Could you check a few things on this model? Use its own coordinates, in mm. Face numbers are marked on the shaded views. A direction names the side the tool comes from. Give positions to 0.01 mm unless a question says otherwise; leave off trailing zeros. Write each loop counter-clockwise with the first axis right and the second up, starting at its lowest first coordinate (ties: lowest second). Pieces come first, ordered by that corner, then holes. Notation, with made-up numbers: (47.25, 56) -> (94.25, 56) arc R17 ccw to (94.25, 69) -> close; hole circle Ø6 at (86.25, 69). An arc over 180 degrees is marked (long way). One line per question, with ' | ' between items.
from build123d import *

# Parameters (mm, degrees)
SKETCH1_W           = 70
SKETCH1_H           = 70
BOSS_EXTRUDE1_DEPTH = 10
CUT_EXTRUDE1_DEPTH  = 51.497524692


with BuildPart() as part:
    # Sketch1 → Boss-Extrude1 (new body)
    with BuildSketch(Plane(origin=(0, 0, 0), x_dir=(1, 0, 0), z_dir=(0, 1, 0))):
        Rectangle(SKETCH1_W, SKETCH1_H)
    extrude(amount=BOSS_EXTRUDE1_DEPTH)

    # Sketch4 → Cut-Extrude1 (cut, through all)
    with BuildSketch(Plane(origin=(0, 10, 0), x_dir=(1, 0, 0), z_dir=(0, 1, 0))):
        with BuildLine():
            Line((-26.870057685, 3.25), (-18.384776311, 3.25))
            ThreePointArc((-18.384776311, 3.25), (-15.134776311, 0), (-18.384776311, -3.25))
            Line((-18.384776311, -3.25), (-26.870057685, -3.25))
            ThreePointArc((-26.870057685, -3.25), (-30.120057685, 0), (-26.870057685, 3.25))
        make_face()
        with BuildLine():
            Line((3.25, 26.870057685), (3.25, 18.384776311))
            ThreePointArc((3.25, 18.384776311), (0, 15.134776311), (-3.25, 18.384776311))
            Line((-3.25, 18.384776311), (-3.25, 26.870057685))
            ThreePointArc((-3.25, 26.870057685), (0, 30.120057685), (3.25, 26.870057685))
        make_face()
        with BuildLine():
            Line((26.870057685, -3.25), (18.384776311, -3.25))
            ThreePointArc((18.384776311, -3.25), (15.134776311, 0), (18.384776311, 3.25))
            Line((18.384776311, 3.25), (26.870057685, 3.25))
            ThreePointArc((26.870057685, 3.25), (30.120057685, 0), (26.870057685, -3.25))
        make_face()
        with BuildLine():
            Line((-3.25, -26.870057685), (-3.25, -18.384776311))
            ThreePointArc((-3.25, -18.384776311), (0, -15.134776311), (3.25, -18.384776311))
            Line((3.25, -18.384776311), (3.25, -26.870057685))
            ThreePointArc((3.25, -26.870057685), (0, -30.120057685), (-3.25, -26.870057685))
        make_face()
    extrude(amount=-CUT_EXTRUDE1_DEPTH, mode=Mode.SUBTRACT)


solid = part.part
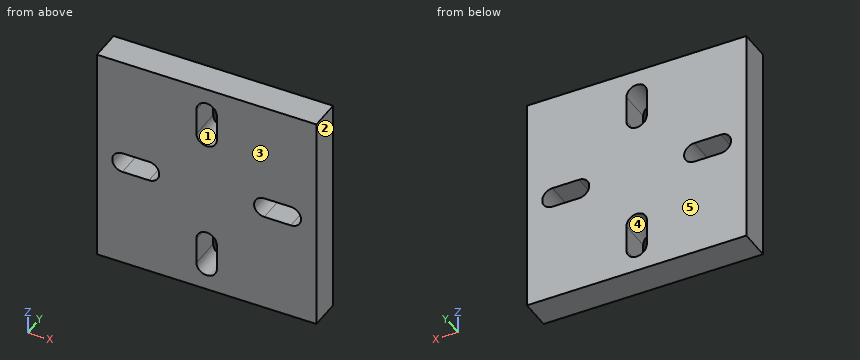
Q1. Imagine slicing it at C-C on y = 4.25. Please give me the cut outline in (x, z), and give its area (3 significant figures).
Answer below:
outline: (-35, -35) -> (35, -35) -> (35, 35) -> (-35, 35) -> close; hole (-26.87, -3.25) -> (-18.38, -3.25) arc R3.25 ccw to (-18.38, 3.25) -> (-26.87, 3.25) arc R3.25 ccw to start; hole (-3.25, -26.87) arc R3.25 ccw to (3.25, -26.87) -> (3.25, -18.38) arc R3.25 ccw to (-3.25, -18.38) -> close; hole (-3.25, 18.38) arc R3.25 ccw to (3.25, 18.38) -> (3.25, 26.87) arc R3.25 ccw to (-3.25, 26.87) -> close; hole (18.38, -3.25) -> (26.87, -3.25) arc R3.25 ccw to (26.87, 3.25) -> (18.38, 3.25) arc R3.25 ccw to start | area: 4,550 mm^2
Q2. If we mould it in two halves opening along X, with no side actions, what happens to the marked faces 1, 2 and 3? For each: +X half, -X half, draft (parallel to the pull), parting line (faces both ways), or undercut.
Answer below:
face 1: undercut | face 2: +X half | face 3: draft
Q3. Imagine slicing it at B-B on x = 0. Please give me the cut outline in (y, z).
Answer below:
outline: (0, -35) -> (10, -35) -> (10, -30.12) -> (0, -30.12) -> close; (0, -15.13) -> (10, -15.13) -> (10, 15.13) -> (0, 15.13) -> close; (0, 30.12) -> (10, 30.12) -> (10, 35) -> (0, 35) -> close
Q4. Imagine slicing it at D-D on z = 17. Please give me the cut outline in (x, y), and give its area (3 significant figures).
Answer below:
outline: (-35, 0) -> (-2.94, 0) -> (-2.94, 10) -> (-35, 10) -> close; (2.94, 0) -> (35, 0) -> (35, 10) -> (2.94, 10) -> close | area: 641 mm^2
Q5. Will this pin go through, and if not, where does the flat tip stop? pin 1 (5 mm diameter, centred on x = -17, z = 8, fed in from -Y).
Answer below:
pin 1: stops at y = 0
Q6. On a 3-axis mill with a long thin cutter (end or side, diameter ignored), from which of +Z, -Z, +X, -X, +Y, -Y can I reach the whole of each face in a straight line? I mean the marked faces 4 and 5. Say none if no direction works.
Answer below:
face 4: +Y, -Y | face 5: +Z, -Z, +X, -X, +Y
Q7. Imagine slicing it at A-A on z = 0. Please give me the cut outline in (x, y), and give its area (3 significant figures).
Answer below:
outline: (-35, 0) -> (-30.12, 0) -> (-30.12, 10) -> (-35, 10) -> close; (-15.13, 0) -> (15.13, 0) -> (15.13, 10) -> (-15.13, 10) -> close; (30.12, 0) -> (35, 0) -> (35, 10) -> (30.12, 10) -> close | area: 400 mm^2
Q8. If I drill on line 1 along X through (y, z) = (2, 21.5); line 2 along Z through (x, y) = (2.5, 5.5), over which ranges is the centre line in solid material (lowest first)?
Answer below:
line 1: x = -35 to -3.25, 3.25 to 35 | line 2: z = -35 to -28.95, -16.31 to 16.31, 28.95 to 35
